from build123d import *

# Parameters (mm, degrees)
BOSS_EXTRUDE1_DEPTH = 3.18
SKETCH3_R           = 6.35
SKETCH3_R_2         = 3.175
SKETCH3_R_3         = 1.65
CUT_EXTRUDE1_DEPTH  = 4.18


with BuildPart() as part:
    # Sketch2 → Boss-Extrude1 (new body)
    with BuildSketch(Plane(origin=(0, 0, 0), x_dir=(1, 0, 0), z_dir=(0, 1, 0))):
        with BuildLine():
            Line((-325, 12.5), (0, 25))
            Line((0, 25), (325, 12.5))
            ThreePointArc((325, 12.5), (337.5, 0), (325, -12.5))
            Line((325, -12.5), (0, -25))
            Line((0, -25), (-325, -12.5))
            ThreePointArc((-325, -12.5), (-337.5, 0), (-325, 12.5))
        make_face()
    extrude(amount=BOSS_EXTRUDE1_DEPTH)

    # Sketch3 → Cut-Extrude1 (cut, through all)
    with BuildSketch(Plane(origin=(0, 3.18, 0), x_dir=(1, 0, 0), z_dir=(0, 1, 0))):
        Circle(SKETCH3_R)
        with Locations((-325, 0)):
            Circle(SKETCH3_R_2)
        with Locations((-217.75, 9.625)):
            Circle(SKETCH3_R_3)
        with Locations((-107.25, -13.875)):
            Circle(SKETCH3_R_3)
        with Locations((325, 0)):
            Circle(SKETCH3_R_2)
        with Locations((-107.25, 13.875)):
            Circle(SKETCH3_R_3)
        with Locations((-217.75, -9.625)):
            Circle(SKETCH3_R_3)
        with Locations((107.25, -13.875)):
            Circle(SKETCH3_R_3)
        with Locations((107.25, 13.875)):
            Circle(SKETCH3_R_3)
        with Locations((217.75, -9.625)):
            Circle(SKETCH3_R_3)
        with Locations((217.75, 9.625)):
            Circle(SKETCH3_R_3)
    extrude(amount=-CUT_EXTRUDE1_DEPTH, mode=Mode.SUBTRACT)


solid = part.part
Read the model definition and answer for the solid it produces. Units are mm, in the model's axes. Give positions to 0.01 mm unless a question says otherwise; leave off trailing zeros. Loops run counter-clockwise (first coordinate to the right, second up) from the corner with the lowest first, then second, coordinate; pieces in that order, holes last. Notation, with made-up numbers: (-39.5, 74.5) - (-28.5, 74.5) arc R17 ccw to (-28.5, 98.5) - close; hole circle Ø10 at (-30, 72.25). An arc over 180 degrees is marked (long way). Answer as CSV lines item,"result". Start each with the question number.
1) Find section B-B (x = -65). Write down the section's boundary in (y, z).
2) Find section A-A (y = 2.5). State how many separate pieces and enclosed holes the cut face has, then the cut area to 3 significant figures.
3) Determine the mould class of faces 1 (the face through (-1.38, 1.61, 6.2)), 2 (the face through (5, 0, 5)), 3 (the face through (160.225, 1.568, -18.838)) for opening direction X: released by +X, released by -X, zero draft, split by the parting line, or undercut.
4) Straight lines are drawn through the part: L1, parallel to Z at x = -325, y = 1.35 (3 decimals); L2, parallel to Z at x = 107.25, y = 2.3 (3 decimals); L3, parallel to X at y = 2, z = 9. For each, find the intervals that lie inside material, in ascending order. Write a range as from..to.
5) Each of these flat-tipped pins is pushed along its axis until it touches: pin 1 Ø2 at (x, z) = (-217.75, -9.625) entering from +Y; pin 2 Ø4.5 at (x, z) = (107.25, -13.875) entering from +Y; pin 3 Ø1.5 at (y, z) = (0.5, 1) entering from -X. Where does it stop, or does it pass through?
Findings below:
1,outline,"(0, -22.5) - (3.18, -22.5) - (3.18, 22.5) - (0, 22.5) - close"
2,separate pieces,"1"
2,enclosed holes,"11"
2,area,"24,600 mm^2"
3,face 1,"undercut"
3,face 2,"zero draft"
3,face 3,"released by +X"
4,L1,"-12.5..-3.175, 3.175..12.5"
4,L2,"-20.875..-15.525, -12.225..12.225, 15.525..20.875"
4,L3,"-333.67..-219.28, -216.22..216.22, 219.28..333.67"
5,pin 1,"through"
5,pin 2,"y = 3.18"
5,pin 3,"x = -337.5"
